The listing builds one solid part. Answer for the finished solid, in the listing's coordinates (mm). A direction names the side the tool comes from. Give positions to 0.01 mm unless a question says otherwise; leave off trailing zeros. Loops run counter-clockwise (first coordinate to the right, second up) from the corner with the lowest first, then second, coordinate; pieces in that order, holes last. Notation, with made-up numbers: (-17, -39.5) - (-4, -39.5) arc R13 ccw to (-4, -33.5) - close; hole circle Ø5 at (47, 40). An arc over 180 degrees is marked (long way). Write item = value, one per line. Start each with the question number.
1) The mould has two halves that part along Y. Classify faces 3 (the cylindrical face through (4.902, -12.032, 23.028)), 4 (the cylindrical face through (-9.967, -3.139, 11.367)), 5 (the flat face through (0, 0, 0)): +Y half, -Y half, draft (parallel to the pull), parting line (faces both ways), or undercut.
2) The part is cut by section B-B on y = -13. Write down the section's boundary in (x, z), plus the area to 3 significant figures.
3) Which of the six approach directions +Z, -Z, +X, -X, +Y, -Y give full straight-line access (tool end or side, diameter ignored) to faces 1 (the cylindrical face through (-9.1, 12.2, 23)), 2 (the flat face through (8, -8, 21))?
4) The part is cut by section D-D on x = 7. State how many separate pieces and enclosed holes the cut face has, plus the area to 3 significant figures.
5) The part is cut by section A-A on x = -14. Write down the section's boundary in (y, z), plus the area to 3 significant figures.
6) Consider probe 1 along Y at (x, z) = (7, 23.25); probe 2 along Y at (x, z) = (-6, 23); probe 3 along Z at (x, y) = (10, -5). Determine where each line is inside the solid, lowest interval first.
7) The part is cut by section C-C on z = 8.5. Write down the section's boundary in (x, y), plus the area to 3 significant figures.
8) Flat-ended cylindrical pins translate along their axes: P1, Ø5, axis at x = -5, z = 6.5, coming from the -Y side; P2, Ø4, axis at x = -9.5, z = 14, coming from the +Y side; P3, Ø8, axis at y = -5.5, z = 20, coming from the -X side. Find the tip coordinate at first contact, or state that the pin passes through.
from build123d import *

# Parameters (mm, degrees)
SKETCH1_R           = 10.45
BOSS_EXTRUDE1_DEPTH = 21
SKETCH2_R           = 17.5
BOSS_EXTRUDE2_DEPTH = 4
SKETCH3_R           = 2.1
CUT_EXTRUDE1_DEPTH  = 36.178118199
FILLET1_R           = 2


with BuildPart() as part:
    # Sketch1 → Boss-Extrude1 (new body)
    with BuildSketch(Plane.XY):
        with Locations(Location((0, 0, 0), (0, 0, 180))):
            Circle(SKETCH1_R)
    extrude(amount=BOSS_EXTRUDE1_DEPTH)

    # Sketch2 → Boss-Extrude2 (add)
    with BuildSketch(Plane.XY.offset(21)):
        Circle(SKETCH2_R)
    extrude(amount=BOSS_EXTRUDE2_DEPTH)

    # Sketch3 → Cut-Extrude1 (cut, through all)
    with BuildSketch(Plane.XY.offset(25)):
        with Locations((14, 0)):
            Circle(SKETCH3_R)
        with Locations((7, -12.124355653)):
            Circle(SKETCH3_R)
        with Locations((-7, -12.124355653)):
            Circle(SKETCH3_R)
        with Locations((-14, 0)):
            Circle(SKETCH3_R)
        with Locations((-7, 12.124355653)):
            Circle(SKETCH3_R)
        with Locations((7, 12.124355653)):
            Circle(SKETCH3_R)
    extrude(amount=-CUT_EXTRUDE1_DEPTH, mode=Mode.SUBTRACT)

    # Fillet1
    fillet1_edges = [part.edges().sort_by_distance(p)[0] for p in [
        (10.45, 0, 0),
    ]]
    fillet(fillet1_edges, radius=FILLET1_R)


solid = part.part
Answer below:
q1.face_3 = undercut
q1.face_4 = parting line
q1.face_5 = draft
q2.outline = (-11.72, 21) - (-8.91, 21) - (-8.91, 25) - (-11.72, 25) - close; (-5.09, 21) - (5.09, 21) - (5.09, 25) - (-5.09, 25) - close; (8.91, 21) - (11.72, 21) - (11.72, 25) - (8.91, 25) - close
q2.area = 63.2 mm2
q3.face_1 = +Z, -Z
q3.face_2 = -Z
q4.separate_pieces = 3
q4.enclosed_holes = 0
q4.area = 418 mm2
q5.outline = (-10.5, 21) - (-2.1, 21) - (-2.1, 25) - (-10.5, 25) - close; (2.1, 21) - (10.5, 21) - (10.5, 25) - (2.1, 25) - close
q5.area = 67.2 mm2
q6.probe_1 = -16.04 to -14.22, -10.02 to 10.02, 14.22 to 16.04
q6.probe_2 = -16.44 to -13.97, -10.28 to 10.28, 13.97 to 16.44
q6.probe_3 = 21 to 25
q7.outline = circle Ø20.9 at (0, 0)
q7.area = 343 mm2
q8.P1 = -10.15
q8.P2 = 7.28
q8.P3 = -17.42
